from build123d import *

# Parameters (mm, degrees)
F0_R     = 11
F1_DEPTH = 4.4
F2_R     = 11
F2_R_2   = 3.25
F3_DEPTH = 1


# Not quite as in the source:
# - a fillet or chamfer that OpenCascade refuses, or shapes differently, is made with other operations: its cross-section is extruded or revolved along the edge and cut away or added


with BuildPart() as f1:
    # F0 (on Top) → F1 (new body)
    with BuildSketch(Plane.XY):
        Circle(F0_R)
        Polygon((4.0383603583, 4.521243813), (5.9346921779, -1.2367007534), (1.8963318196, -5.7579445664), (-4.0383603583, -4.521243813), (-5.9346921779, 1.2367007534), (-1.8963318196, 5.7579445664), align=None, mode=Mode.SUBTRACT)
    extrude(amount=F1_DEPTH)

    # F2 (on face) → F3 (join)
    with BuildSketch(Plane(origin=(0, 0, 0), x_dir=(1, 0, 0), z_dir=(0, 0, -1))):
        Circle(F2_R)
        Circle(F2_R_2, mode=Mode.SUBTRACT)
    extrude(amount=F3_DEPTH)

    # F4: fillet of radius 5 on 1 edges, made by hand

    # F4_s1 → F4_t2 (revolve, cut)
    with BuildSketch(Plane.XZ):
        with BuildLine():
            ThreePointArc((11, -0.6), (9.5355339059, 2.9355339059), (6, 4.4))
            Line((6, 4.4), (11, 4.4))
            Line((11, 4.4), (11, -0.6))
        make_face()
    revolve(axis=Axis((0, 0, 4.4), (0, 0, 1)), mode=Mode.SUBTRACT)


solid = f1.part
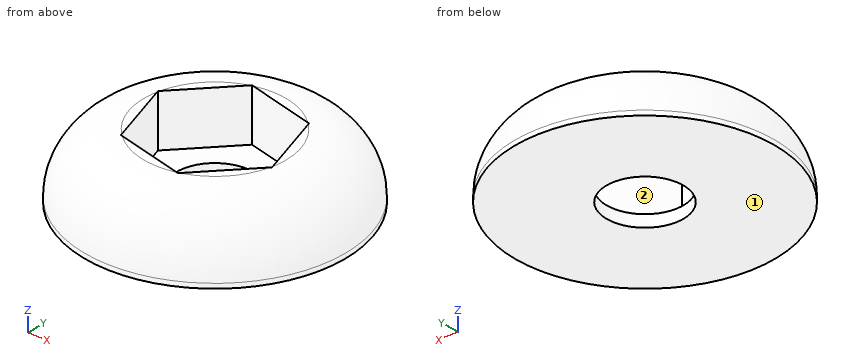
Read the model definition and answer for the solid it produces. Units are mm, in the model's axes. Face numbers are marked on the shaded views. Coordinates: 2 decimals unless noted, no trailing zeros. Loops run counter-clockwise (first coordinate to the right, second up) from the corner with the lowest first, then second, coordinate; pieces in that order, holes last.
Q1. Each of these flat-tipped pins is pushed along its axis until it touches: pin 1 Ø1.5 at (x, z) = (-7, 0) entering from -Y; pin 2 Ø2 at (y, z) = (-7.5, 1.5) entering from +X; pin 3 Ø1.5 at (y, z) = (-1.5, 3) entering from +X; pin 4 Ø3.5 at (x, y) = (-1, -1) entering from +Z. Where does it stop, or does it pass through?
Q2. The part is cut by section C-C on y = 0. Write down the section's boundary in (x, z), and give its area (3 significant figures).
Q3. The part is cut by section A-A on z = 3.1. Write down the section's boundary in (x, y), and give its area (3 significant figures).
Q4. The part is cut by section B-B on x = 0. Write down the section's boundary in (y, z), and give its area (3 significant figures).
Q5. Consider probe 1 along X at (y, z) = (0, -0.75); probe 2 along Z at (x, y) = (5.25, -1). Determine where each line is inside the solid, lowest interval first.
Q6. The mould has two halves that part along Y. Classify the marked faces 1 and 2: +Y half, -Y half, draft (parallel to the pull), parting line (faces both ways), or undercut.
Results below:
1. pin 1: stops at y = -9.02
1. pin 2: stops at x = 8.44
1. pin 3: stops at x = 10.01
1. pin 4: passes through
2. outline: (-11, -1) - (-3.25, -1) - (-3.25, 0) - (-5.53, 0) - (-5.53, 4.4) - (-6, 4.4) arc R5 ccw to (-11, -0.6) - close; (3.25, -1) - (11, -1) - (11, -0.6) arc R5 ccw to (6, 4.4) - (5.53, 4.4) - (5.53, 0) - (3.25, 0) - close
2. area: 52.9 mm2
3. outline: circle Ø18.73 at (0, 0); hole (-5.93, 1.24) - (-4.04, -4.52) - (1.9, -5.76) - (5.93, -1.24) - (4.04, 4.52) - (-1.9, 5.76) - close
3. area: 180 mm2
4. outline: (-11, -1) - (-3.25, -1) - (-3.25, 0) - (-5.36, 0) - (-5.36, 4.4) - (-6, 4.4) arc R5 ccw to (-11, -0.6) - close; (3.25, -1) - (11, -1) - (11, -0.6) arc R5 ccw to (6, 4.4) - (5.36, 4.4) - (5.36, 0) - (3.25, 0) - close
4. area: 54.4 mm2
5. probe 1: x = -11 to -3.25, 3.25 to 11
5. probe 2: z = -1 to 0
6. face 1: draft
6. face 2: undercut
